Design review of the part built by this model. Coordinates are the model's own, in mm. Coordinates: 2 decimals unless noted, no trailing zeros. Loops run counter-clockwise (first coordinate to the right, second up) from the corner with the lowest first, then second, coordinate; pieces in that order, holes last.
Q1. Add section A-A on z = 0. Give the boundary of the cut face in (x, y) (3 decimals), and give its area (3 significant figures).
Q2. Add section B-B on x = 0. Give the boundary of the cut face in (y, z) (3 decimals), and give its area (3 significant figures).
Q3. Wall thickness on probe 1 along X at (y, z) = (1.25, 0); probe 2 along Z at (x, y) = (-34, 0.3): over which ranges is each line inside the solid? List them lowest first.
Q4. Add section D-D on z = -29. Give the boundary of the cut face in (x, y) (3 decimals).
Q5. Add section C-C on y = 1.65. Give the number of separate pieces and of enclosed holes in the cut face, and give its area (3 significant figures).
Q6. For P1, Ø1, axis at y = 2, z = -19, coming from the +X side; P2, Ø1, axis at y = 1.5, z = -19.5, coming from the +X side, all flat-tipped, find the tip position at first contact; note any pin that passes through.
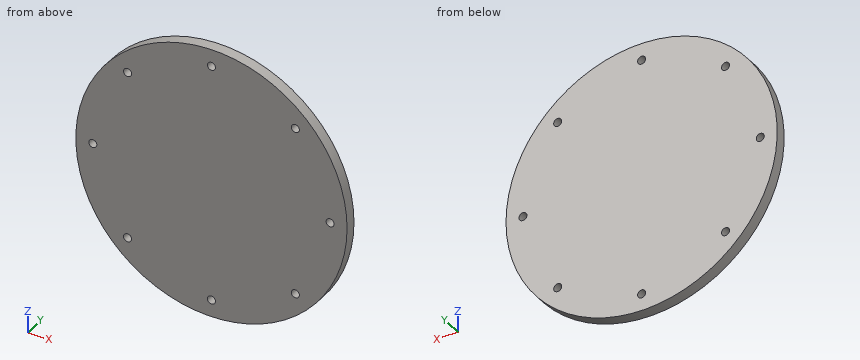
```python
from build123d import *

# Parameters (mm, degrees)
SKETCH1_R                 = 38.1
BOSS_EXTRUDE1_DEPTH       = 3.175
TAP_DRILL_FOR_4_40_TAP1_D = 2.2606
CIRPATTERN1_COUNT         = 8


with BuildPart() as part:
    # Sketch1 → Boss-Extrude1 (new body)
    with BuildSketch(Plane(origin=(0, 0, 0), x_dir=(1, 0, 0), z_dir=(0, 1, 0))):
        Circle(SKETCH1_R)
    extrude(amount=BOSS_EXTRUDE1_DEPTH)

    # Tap Drill for #4-40 Tap1 (through all)
    with Locations(Plane(origin=(0, 0, 0), x_dir=(-1, 0, 0), z_dir=(0, -1, 0))):
        with Locations((0, -33.3375)):
            tap_drill_for_4_40_tap1 = Hole(TAP_DRILL_FOR_4_40_TAP1_D / 2)

    # CirPattern1: Tap Drill for #4-40 Tap1 ×8 about axis
    cirpattern1_axis = Axis((0, 0, 0), (0, 1, 0))
    for i in range(1, CIRPATTERN1_COUNT):
        add(tap_drill_for_4_40_tap1.rotate(cirpattern1_axis, i * 360 / CIRPATTERN1_COUNT), mode=Mode.SUBTRACT)


solid = part.part
```
Entries:
1. outline: (-38.1, 0) - (-34.468, 0) - (-34.468, 3.175) - (-38.1, 3.175) - close; (-32.207, 0) - (32.207, 0) - (32.207, 3.175) - (-32.207, 3.175) - close; (34.468, 0) - (38.1, 0) - (38.1, 3.175) - (34.468, 3.175) - close
1. area: 228 mm2
2. outline: (0, -38.1) - (3.175, -38.1) - (3.175, -34.468) - (0, -34.468) - close; (0, -32.207) - (3.175, -32.207) - (3.175, 32.207) - (0, 32.207) - close; (0, 34.468) - (3.175, 34.468) - (3.175, 38.1) - (0, 38.1) - close
2. area: 228 mm2
3. probe 1: x = -38.1 to -34.47, -32.21 to 32.21, 34.47 to 38.1
3. probe 2: z = -17.19 to -0.92, 0.92 to 17.19
4. outline: (-24.711, 0) - (24.711, 0) - (24.711, 3.175) - (-24.711, 3.175) - close
5. separate pieces: 1
5. enclosed holes: 8
5. area: 4,530 mm2
6. P1: stops at x = 33.31
6. P2: stops at x = 33.02
